Part model, mm, in its own coordinate system. A direction names the side the tool comes from. Round coordinates to 2 decimals unless told otherwise and drop trailing zeros. Write each loop counter-clockwise with the first axis right and the second up, starting at its lowest first coordinate (ties: lowest second). Pieces come first, ordered by that corner, then holes. Notation, with made-up numbers: M 55,55 L 63,55 A28 ccw 63,84 Z; hole C 50,-16.5 d3. An arc over 180 degrees is marked long. Use one line per item in the form item = value. Start each with the question number.
Item 1: Cut at A-A, the plane y = 0. Give the cut face in (x, z), then the cut area to 3 significant figures.
Item 2: Mould opens along Y. For faces 3 (the face through (-5.719, -0.217, 0.474)), 4 (the face through (-1.438, -0.748, 1.47)), 5 (the face through (0, -2, 0)) say: +Y half, -Y half, draft (parallel to the pull), parting line (faces both ways), or undercut.
Item 3: Cut at C-C, the plane x = -0.5. Give the cut face in (y, z), then the cut area to 3 significant figures.
Item 4: Probe L1, parallel to X at y = 0, z = 2.2; L2, parallel to X at y = -1.25, z = 2.4; L3, parallel to Z at x = 3.75, y = 0. List the from-to ranges inside material, lowest first.
Item 5: Cut at B-B, the plane z = 2.25. Give the cut face in (x, y).
Item 6: Cut at D-D, the plane z = 1.45. Give the cut face in (x, y), then the cut area to 3 significant figures.
Item 7: Flat gauge pins, fed straight in: pin 1 Ø1 at (x, z) = (1, 2) entering from -Y; pin 2 Ø1 at (x, y) = (6, -0.5) entering from +Z. Where does each tip first touch, or does it go through?
Item 8: Which spindle directions (+Z, -Z, +X, -X, +Y, -Y) get a long thin tool onto all of the face, cutting with end or side? Do faces 1 (the face through (-8, 0, 1)), 2 (the face through (5.72, -0.13, 0.46)). Say none if no direction does.
Solid Edge part; units mm, degrees
sketch "Sketch1" plane through (0, 0, 0) normal (0, 0, 1) x (1, 0, 0)
  line L0 (3.5, 2.0207) -> (0, 4.0415)
  line L1 (0, 4.0415) -> (-3.5, 2.0207)
  line L2 (-3.5, 2.0207) -> (-3.5, -2.0207)
  line L3 (-3.5, -2.0207) -> (0, -4.0415)
  line L4 (0, -4.0415) -> (3.5, -2.0207)
  line L5 (3.5, -2.0207) -> (3.5, 2.0207)
extrude "Protrusion1" add sketch "Sketch1" along normal blind 2.9
hole "Otwór_1" at (0, 0, 2.9) direction (0, 0, -1) diameter 3.242 end up to next
sketch "Sketch2" plane through (3.5, 0, 1.45) normal (1, 0, 0) x (0, 1, 0)
  circle A0 centre (0, 0) radius 1
extrude "Wyciągnięcie_2" add sketch "Sketch2" along normal blind 4.5
mirror "Mirror1" about plane through (0, 4.0415, 2.9) normal (-1, 0, 0) of "Wyciągnięcie_2"
Model answer:
q1.outline = M -8,0.45 L -3.5,0.45 L -3.5,0 L -1.62,0 L -1.62,2.9 L -3.5,2.9 L -3.5,2.45 L -8,2.45 Z; M 1.62,0 L 3.5,0 L 3.5,0.45 L 8,0.45 L 8,2.45 L 3.5,2.45 L 3.5,2.9 L 1.62,2.9 Z
q1.area = 28.9 mm²
q2.face_3 = parting line
q2.face_4 = undercut
q2.face_5 = draft
q3.outline = M -3.75,0 L -1.54,0 L -1.54,2.9 L -3.75,2.9 Z; M 1.54,0 L 3.75,0 L 3.75,2.9 L 1.54,2.9 Z
q3.area = 12.8 mm²
q4.L1 = -8 to -1.62, 1.62 to 8
q4.L2 = -3.5 to -1.03, 1.03 to 3.5
q4.L3 = 0.45 to 2.45
q5.outline = M -8,-0.6 L -3.5,-0.6 L -3.5,-2.02 L 0,-4.04 L 3.5,-2.02 L 3.5,-0.6 L 8,-0.6 L 8,0.6 L 3.5,0.6 L 3.5,2.02 L 0,4.04 L -3.5,2.02 L -3.5,0.6 L -8,0.6 Z; hole C 0,0 d3.24
q6.outline = M -8,-1 L -3.5,-1 L -3.5,-2.02 L 0,-4.04 L 3.5,-2.02 L 3.5,-1 L 8,-1 L 8,1 L 3.5,1 L 3.5,2.02 L 0,4.04 L -3.5,2.02 L -3.5,1 L -8,1 Z; hole C 0,0 d3.24
q6.area = 52.2 mm²
q7.pin_1 = -3.75
q7.pin_2 = 2.45
q8.face_1 = +Z, -Z, -X, +Y, -Y
q8.face_2 = +X
